Autodesk Inventor part; units mm, degrees
ref_plane "YZ Plane" through (0, 0, 0) normal (1, 0, 0) x (0, 1, 0)
ref_plane "XZ Plane" through (0, 0, 0) normal (0, 1, 0) x (-1, 0, 0)
ref_plane "XY Plane" through (0, 0, 0) normal (0, 0, 1) x (1, 0, 0)
sketch "Sketch1" plane through (0, 0, 0) normal (0, 0, 1) x (1, 0, 0)
  line L0 (2.5847, -1.4923) -> (1.3748, -0.7938)
  arc A0 (2.5847, -1.4923) -> (0, -2.9845) centre (0, 0) ccw
  arc A1 (1.3748, -0.7938) -> (0, -1.5875) centre (0, 0) ccw
  arc A2 (1.3748, -0.7938) -> (0, -1.5875) centre (0, 0) ccw
  line L1 (0, -1.5875) -> (16.8049, -1.5875)
  line L2 (16.8049, -2.9845) -> (0, -2.9845)
  arc A3 (2.5847, -1.4923) -> (0, -2.9845) centre (0, 0) ccw
  line L3 (2.5847, -1.4923) -> (1.3748, -0.7938)
  line L4 (19.05, -1.5875) -> (16.8049, -1.5875)
  line L5 (19.05, -2.9845) -> (16.8049, -2.9845)
  line L6 (19.05, -1.5875) -> (19.05, -2.9845)
  point P0 (0, 0)
  point P1 (15.875, -2.9845)
extrude "Extrusion1" add sketch "Sketch1" against normal blind 63.5
sketch "Sketch2" plane through (0, -2.9845, 0) normal (0, -1, 0) x (1, 0, 0)
  line L0 (19.05, -23.1549) -> (19.05, -14.9451)
  line L1 (19.05, -14.9451) -> (16.8049, -12.7)
  line L2 (16.8049, -12.7) -> (19.05, -10.4549)
  line L3 (19.05, -10.4549) -> (19.05, -2.2451)
  line L4 (19.05, -2.2451) -> (16.8049, 0)
  line L5 (0, 0) -> (16.8049, 0)
  line L6 (0, -7.1247) -> (0, 0)
  line L7 (5.8525, -7.1247) -> (-2.9845, -7.1247)
  line L8 (5.8525, -23.8125) -> (5.8525, -7.1247)
  line L9 (5.8525, -23.8125) -> (-2.9845, -23.8125)
  line L10 (0, -39.6875) -> (0, -23.8125)
  line L11 (5.8525, -39.6875) -> (-2.9845, -39.6875)
  line L12 (5.8525, -56.3753) -> (5.8525, -39.6875)
  line L13 (-2.9845, -56.3753) -> (5.8525, -56.3753)
  line L14 (0, -63.5) -> (0, -56.3753)
  line L15 (16.8049, -63.5) -> (0, -63.5)
  line L16 (16.8049, -63.5) -> (19.05, -61.2549)
  line L17 (19.05, -61.2549) -> (19.05, -53.0451)
  line L18 (19.05, -53.0451) -> (16.8049, -50.8)
  line L19 (16.8049, -50.8) -> (19.05, -48.5549)
  line L20 (19.05, -48.5549) -> (19.05, -40.3451)
  line L21 (19.05, -40.3451) -> (16.8049, -38.1)
  line L22 (16.8049, -38.1) -> (19.05, -35.8549)
  line L23 (19.05, -35.8549) -> (19.05, -27.6451)
  line L24 (19.05, -27.6451) -> (16.8049, -25.4)
  line L25 (16.8049, -25.4) -> (19.05, -23.1549)
  line L26 (15.0114, -42.1386) -> (15.0114, -46.7614)
  line L27 (15.0114, -46.7614) -> (10.3886, -46.7614)
  line L28 (10.3886, -46.7614) -> (10.3886, -42.1386)
  line L29 (10.3886, -42.1386) -> (15.0114, -42.1386)
  line L30 (15.0114, -29.4386) -> (15.0114, -34.0614)
  line L31 (15.0114, -34.0614) -> (10.3886, -34.0614)
  line L32 (10.3886, -34.0614) -> (10.3886, -29.4386)
  line L33 (10.3886, -29.4386) -> (15.0114, -29.4386)
  line L34 (15.0114, -16.7386) -> (15.0114, -21.3614)
  line L35 (15.0114, -21.3614) -> (10.3886, -21.3614)
  line L36 (10.3886, -21.3614) -> (10.3886, -16.7386)
  line L37 (10.3886, -16.7386) -> (15.0114, -16.7386)
  line L38 (15.0114, -4.0386) -> (15.0114, -8.6614)
  line L39 (15.0114, -8.6614) -> (10.3886, -8.6614)
  line L40 (10.3886, -8.6614) -> (10.3886, -4.0386)
  line L41 (10.3886, -4.0386) -> (15.0114, -4.0386)
  line L42 (15.0114, -54.8386) -> (15.0114, -59.4614)
  line L43 (15.0114, -59.4614) -> (10.3886, -59.4614)
  line L44 (10.3886, -59.4614) -> (10.3886, -54.8386)
  line L45 (10.3886, -54.8386) -> (15.0114, -54.8386)
  line L46 (-2.9845, 0) -> (-2.9845, -63.5)
  line L47 (19.05, -53.0451) -> (19.05, -48.5549)
  line L48 (19.05, -40.3451) -> (19.05, -35.8549)
  line L49 (19.05, -27.6451) -> (19.05, -23.1549)
  line L50 (19.05, -14.9451) -> (19.05, -10.4549)
  line L51 (0, 0) -> (16.8049, 0)
  line L52 (16.8049, -63.5) -> (19.05, -63.5)
  line L53 (19.05, -63.5) -> (19.05, -61.2549)
  line L54 (19.05, -2.2451) -> (19.05, 0)
  line L55 (19.05, 0) -> (16.8049, 0)
  line L56 (16.8049, -63.5) -> (19.05, -61.2549)
  line L57 (19.05, -2.2451) -> (16.8049, 0)
  point P0 (15.875, -31.75)
extrude "Extrusion2" cut sketch "Sketch2" against normal blind 6.35 contours L49 L24 L25 | L1 L2 L50 | L48 L21 L22 | L4 L55 L54 | L47 L18 L19 | L7 L8 L9 L46 | L53 L52 L16 | L11 L12 L13 L46 | L26 L27 L28 L29 | L30 L31 L32 L33 | L34 L35 L36 L37 | L38 L39 L40 L41 | L42 L43 L44 L45
sketch "Sketch3" plane through (0, -2.9845, 0) normal (0, -1, 0) x (1, 0, 0)
  line L0 (15.0114, -8.6614) -> (10.3886, -8.6614)
  circle A0 centre (12.7, -6.35) radius 2.3114
surface extrude "ExtrusionSrf1" sketch "Sketch3" against normal up to surface (1.397 mm away) shown no curves A0
pattern_linear "Rectangular Pattern1" count 5 spacing 12.7 along (0, 0, -1) of "ExtrusionSrf1"
properties part number "275-1272"
The model under review builds one solid part; all positions refer to its coordinate system, in mm. A direction names the side the tool comes from. Coordinates: 2 decimals unless noted, no trailing zeros. Write each loop counter-clockwise with the first axis right and the second up, starting at its lowest first coordinate (ties: lowest second). Pieces come first, ordered by that corner, then holes. Notation, with made-up numbers: (-11.75, -24) -> (5.25, -24) arc R21 cw to (5.25, -11) -> close; hole circle Ø8 at (13, 63.25). An arc over 180 degrees is marked (long way). One line per item, written item: value. Start each with the question number.
Q1. To check wall thickness, follow probe 1 along Z at (x, y) = (2, 0.5); probe 2 along Z at (x, y) = (13.5, -2); probe 3 along X at (y, z) = (-2, -45.5). State the ranges of each line that lie inside material, in increasing order.
Q2. Clearance check with flat-ended pins moving along their axes: P1, Ø1.5, axis at y = -0.5, z = -34, coming from the -X side; P2, Ø1.5, axis at y = -1.5, z = -25.5, coming from the -X side; P3, Ø1.1, axis at y = -2, z = -58, coming from the -X side. State where each tip first meets the part, or that it passes through.
Q3. The part is to be moulded in two halves that separate along Z. For faces 5 (the face through (-1.396, 2.638, -31.639)), 6 (the face through (17.912, -2.296, -62.393)), 7 (the face through (13, -2, -4.039)), 8 (the face through (13, -2, -54.839)), say which applies: +Z half, -Z half, draft (parallel to the pull), parting line (faces both ways), or undercut.
Q4. Add section B-B, the plane x = 12.25. Give the boundary of the cut face in (y, z), then the cut area to 3 significant figures.
Q5. Add section A-A, the plane z = -6. Give the boundary of the cut face in (x, y).
Q6. Add section D-D, the plane y = 2.4. Give the boundary of the cut face in (x, z).
Q7. For faces 1 (the face through (13, -2, -16.739)), 2 (the face through (17.943, -2.296, -26.538)), 3 (the face through (5.852, -2, -48)), 4 (the face through (-1.396, 2.638, -3.512)), list the 3-axis set-ups (+Z, -Z, +X, -X, +Y, -Y) from which the entire face can be reached by the end or side of a thin tool; tool diameter is ignored.
Q8. Add section C-C, the plane x = 4.25. Give the boundary of the cut face in (y, z).
Response:
1. probe 1: -63.5 to -56.38, -39.69 to -23.81, -7.12 to 0
1. probe 2: -63.5 to -59.46, -54.84 to -46.76, -42.14 to -34.06, -29.44 to -21.36, -16.74 to -8.66, -4.04 to 0
1. probe 3: 5.85 to 10.39, 15.01 to 19.05
2. P1: x = -2.98
2. P2: x = -2.89
2. P3: x = -2.61
3. face 5: draft
3. face 6: -Z half
3. face 7: undercut
3. face 8: undercut
4. outline: (-2.98, -63.5) -> (-1.59, -63.5) -> (-1.59, -59.46) -> (-2.98, -59.46) -> close; (-2.98, -54.84) -> (-1.59, -54.84) -> (-1.59, -46.76) -> (-2.98, -46.76) -> close; (-2.98, -42.14) -> (-1.59, -42.14) -> (-1.59, -34.06) -> (-2.98, -34.06) -> close; (-2.98, -29.44) -> (-1.59, -29.44) -> (-1.59, -21.36) -> (-2.98, -21.36) -> close; (-2.98, -16.74) -> (-1.59, -16.74) -> (-1.59, -8.66) -> (-2.98, -8.66) -> close; (-2.98, -4.04) -> (-1.59, -4.04) -> (-1.59, 0) -> (-2.98, 0) -> close
4. area: 56.4 mm²
5. outline: (0, -2.98) -> (10.39, -2.98) -> (10.39, -1.59) -> (0, -1.59) arc R1.59 cw (long way) to (1.37, -0.79) -> (2.58, -1.49) arc R2.98 ccw (long way) to start; (15.01, -2.98) -> (19.05, -2.98) -> (19.05, -1.59) -> (15.01, -1.59) -> close
6. outline: (-1.77, -63.5) -> (1.77, -63.5) -> (1.77, -56.38) -> (-1.77, -56.38) -> close; (-1.77, -39.69) -> (1.77, -39.69) -> (1.77, -23.81) -> (-1.77, -23.81) -> close; (-1.77, -7.12) -> (1.77, -7.12) -> (1.77, 0) -> (-1.77, 0) -> close
7. face 1: +Y, -Y
7. face 2: +X, +Y, -Y
7. face 3: -X, +Y, -Y
7. face 4: +Z, -Z
8. outline: (-2.98, -63.5) -> (-1.59, -63.5) -> (-1.59, -56.38) -> (-2.98, -56.38) -> close; (-2.98, -39.69) -> (-1.59, -39.69) -> (-1.59, -23.81) -> (-2.98, -23.81) -> close; (-2.98, -7.12) -> (-1.59, -7.12) -> (-1.59, 0) -> (-2.98, 0) -> close
